from build123d import *

# Parameters (mm, degrees)
SKETCH1_W           = 28
SKETCH1_H           = 20
BOSS_EXTRUDE1_DEPTH = 3.3
BOSS_EXTRUDE2_DEPTH = 10
SKETCH3_W           = 24.7
SKETCH3_H           = 13.4
CUT_EXTRUDE1_DEPTH  = 24.7


with BuildPart() as part:
    # Sketch1 → Boss-Extrude1 (new body)
    with BuildSketch(Plane(origin=(0, 0, 0), x_dir=(0, 0, -1), z_dir=(1, 0, 0))):
        with Locations((14, 10)):
            Rectangle(SKETCH1_W, SKETCH1_H)
        with BuildLine():
            Line((12.5, 13.28), (17.7, 13.28))
            ThreePointArc((17.7, 13.28), (20.7, 10.28), (17.7, 7.28))
            Line((17.7, 7.28), (12.5, 7.28))
            ThreePointArc((12.5, 7.28), (9.5, 10.28), (12.5, 13.28))
        make_face(mode=Mode.SUBTRACT)
    boss_extrude1 = extrude(amount=BOSS_EXTRUDE1_DEPTH)

    # Mirror1: Boss-Extrude1 across plane
    add(boss_extrude1.mirror(Plane(origin=(14, 0, -14), x_dir=(0.707106781, 0, 0.707106781), z_dir=(-0.707106781, 0, 0.707106781))))

    # Sketch2 → Boss-Extrude2 (add, symmetric)
    with BuildSketch(Plane(origin=(0, 10, 0), x_dir=(1, 0, 0), z_dir=(0, 1, 0))):
        Polygon((3.3, 0), (6, 0), (6, 4.7), (23.3, 22), (28, 22), (28, 24.7), (3.3, 24.7), align=None)
    extrude(amount=BOSS_EXTRUDE2_DEPTH, both=True)

    # Sketch3 → Cut-Extrude1 (cut)
    with BuildSketch(Plane.XY):
        with Locations((15.65, 10)):
            Rectangle(SKETCH3_W, SKETCH3_H)
    extrude(amount=-CUT_EXTRUDE1_DEPTH, mode=Mode.SUBTRACT)


solid = part.part
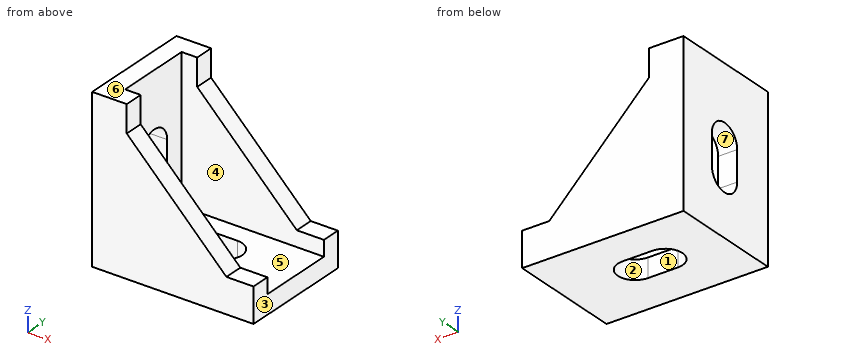
CAD build for the part. Positions are in the model's coordinates, mm. Face numbers are marked on the shaded views. A direction names the side the tool comes from. Coordinates: 2 decimals unless noted, no trailing zeros. Order: outer loops, then holes, each group sorted by start corner. A loop starts at its lowest first (then second) coordinate and runs counter-clockwise, first axis right, second up. Notation, with made-up numbers: (-15.75, 83) -> (-10.75, 83) arc R28 cw to (-10.75, 119) -> close; hole circle Ø9 at (70, 86.25). An arc over 180 degrees is marked (long way). Answer in a Markdown table with one row per item.
1) Band-saw the part on B-B (z = -15). List the corners of the cut face in (x, y).
Check values:
| item | result |
|---|---|
| outline | (0, 0) -> (16.3, 0) -> (16.3, 3.3) -> (3.3, 3.3) -> (3.3, 7.28) -> (0, 7.28) -> close; (0, 13.28) -> (3.3, 13.28) -> (3.3, 16.7) -> (16.3, 16.7) -> (16.3, 20) -> (0, 20) -> close |
2) Flat gauge pins, fed straight in: P1, Ø6, axis at y = 11.5, z = -10.5, coming from the +X side; P2, Ø12.5, axis at x = 13, z = -11, coming from the -Y side; P3, Ø4, axis at x = 19.5, y = 13, coming from the +Z side; P4, Ø2.5, axis at x = 25.5, y = 1.5, coming from the +Z side. Where does each tip first touch, or does it go through?
Check values:
| item | result |
|---|---|
| P1 | x = 3.3 |
| P2 | y = 0 |
| P3 | z = -24.7 |
| P4 | z = -22 |
3) Mould opens along X. For the marked faces 1, 2, 3 and 4 say: pulls with the +X half, pulls with the -X half, needs draft (parallel to the pull), parting line crosses it, or undercut.
Check values:
| item | result |
|---|---|
| face 1 | undercut |
| face 2 | undercut |
| face 3 | pulls with the +X half |
| face 4 | needs draft |
4) Band-saw the part on A-A (x = 14.75). List the corners of the cut face in (y, z).
Check values:
| item | result |
|---|---|
| outline | (0, -28) -> (7.28, -28) -> (7.28, -24.7) -> (3.3, -24.7) -> (3.3, -13.45) -> (0, -13.45) -> close; (13.28, -28) -> (20, -28) -> (20, -13.45) -> (16.7, -13.45) -> (16.7, -24.7) -> (13.28, -24.7) -> close |
5) Band-saw the part on D-D (x = 24). List the corners of the cut face in (y, z), and give its area (3 significant figures).
Check values:
| item | result |
|---|---|
| outline | (0, -28) -> (20, -28) -> (20, -22) -> (16.7, -22) -> (16.7, -24.7) -> (3.3, -24.7) -> (3.3, -22) -> (0, -22) -> close |
| area | 83.8 mm2 |
6) Which spindle directions (+Z, -Z, +X, -X, +Y, -Y) get a long thin tool onto all of the face, cutting with end or side? Do the marked faces 5, 6 and 7. Say none if no direction does.
Check values:
| item | result |
|---|---|
| face 5 | +Z, +X |
| face 6 | +Z, +X, -X, +Y, -Y |
| face 7 | +X, -X |
7) Drill centre lines: line 1 (Y direction, x = 4.5, z = -7.5); line 2 (Z direction, x = 7, y = 10.5); line 3 (X direction, y = 14.5, z = -24.25). Where is each one in solid material? Low to high.
Check values:
| item | result |
|---|---|
| line 1 | 0 to 3.3, 16.7 to 20 |
| line 2 | -28 to -24.7 |
| line 3 | 0 to 3.3 |
8) Band-saw the part on C-C (y = 10.28). List the corners of the cut face in (x, z).
Check values:
| item | result |
|---|---|
| outline | (0, -28) -> (7.3, -28) -> (7.3, -24.7) -> (3.3, -24.7) -> (3.3, -20.7) -> (0, -20.7) -> close; (0, -9.5) -> (3.3, -9.5) -> (3.3, 0) -> (0, 0) -> close; (18.5, -28) -> (28, -28) -> (28, -24.7) -> (18.5, -24.7) -> close |
